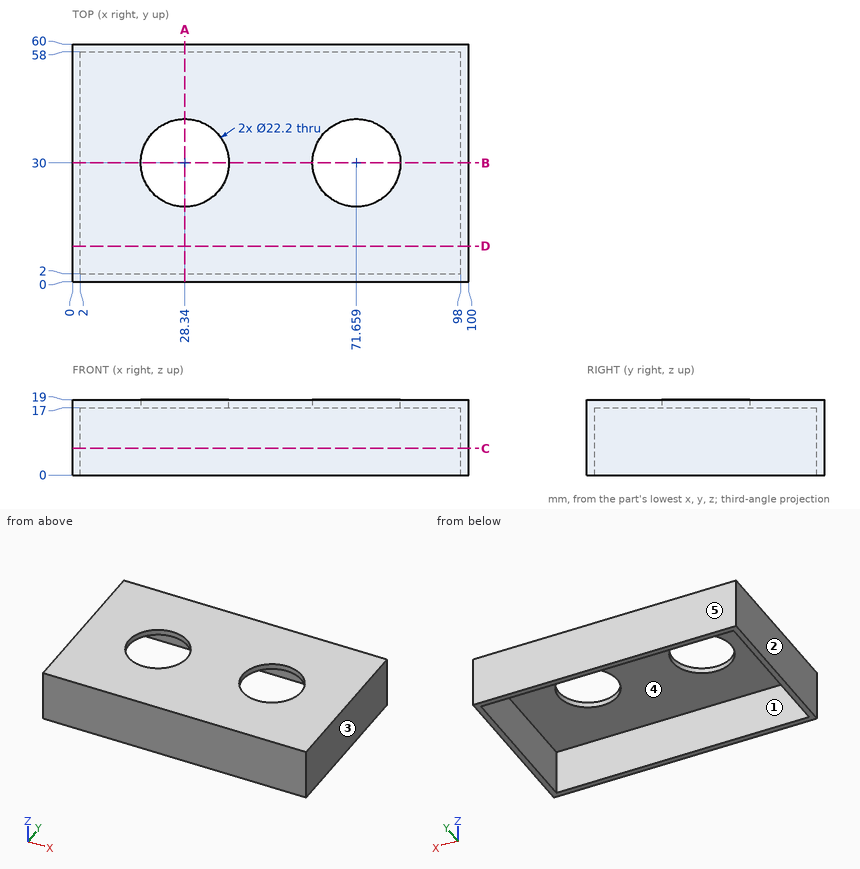
Input: dimensioned drawing with shaded views. Units: mm. Origin: part minimum x, y, z. A direction names the side the tool comes from. Coordinates: 2 decimals unless noted, no trailing zeros. Loops run counter-clockwise (first coordinate to the right, second up) from the corner with the lowest first, then second, coordinate; pieces in that order, holes last. Notation, with made-up numbers: M 56,-13.75 L 105,-13.75 A21 ccw 105,21.25 Z; hole C 23.5,78 d5. An arc over 180 degrees is marked long. One line per item, written item: value. Start each with the question number.
1) Pin query (flat end, axial travel): P1, Ø2, axis at x = 62, y = 45.5, coming from the -Z side. Return the tip coordinate at first contact, or that it passes through.
2) Reachability of the marked faces 1 and 2 from +Z, -Z, +X, -X, +Y, -Y: full face, straight path, thin tool, end or side. Return the list, or none.
3) Cut plane C-C (z = 6.75). Return loops of the section in (x, y), then the cut area to 3 significant figures.
4) Cut plane D-D (y = 9). Return loops of the section in (x, z), then the cut area to 3 significant figures.
5) Cut plane B-B (y = 30). Return loops of the section in (x, z), then the cut area to 3 significant figures.
6) Material intervals for L1, parallel to X at y = 30, z = 18.65; L2, parallel to X at y = 11, z = 15.25; L3, parallel to Y at x = 94.5, z = 3.25, sorted ascending. Write a range as from..to.
7) Draft query along X for the marked faces 3, 4 and 5. Return one class per face: released by +X, released by -X, zero draft, split by the parting line, or undercut.
8) Cut plane A-A (x = 28.34). Return loops of the section in (y, z), then the cut area to 3 significant figures.
Evaluation:
1. P1: z = 17
2. face 1: -Z
2. face 2: +Z, -Z, -X, +Y, -Y
3. outline: M 0,0 L 100,0 L 100,60 L 0,60 Z; hole M 2,2 L 98,2 L 98,58 L 2,58 Z
3. area: 624 mm^2
4. outline: M 0,0 L 2,0 L 2,17 L 98,17 L 98,0 L 100,0 L 100,19 L 0,19 Z
4. area: 268 mm^2
5. outline: M 0,0 L 2,0 L 2,17 L 17.24,17 L 17.24,19 L 0,19 Z; M 39.44,17 L 60.56,17 L 60.56,19 L 39.44,19 Z; M 82.76,17 L 98,17 L 98,0 L 100,0 L 100,19 L 82.76,19 Z
5. area: 179 mm^2
6. L1: 0..17.24, 39.44..60.56, 82.76..100
6. L2: 0..2, 98..100
6. L3: 0..2, 58..60
7. face 3: released by +X
7. face 4: undercut
7. face 5: zero draft
8. outline: M 0,0 L 2,0 L 2,17 L 18.9,17 L 18.9,19 L 0,19 Z; M 41.1,17 L 58,17 L 58,0 L 60,0 L 60,19 L 41.1,19 Z
8. area: 144 mm^2
